Model file for the job. Use its own axes, mm. Face numbers are marked on the shaded views. A direction names the side the tool comes from. Give positions to 0.01 mm unless a question says otherwise; leave off trailing zeros. Write each loop counter-clockwise with the first axis right and the second up, starting at its lowest first coordinate (ties: lowest second). Pieces come first, ordered by that corner, then holes. Notation, with made-up numbers: (38.5, -28.75) - (60.5, -28.75) arc R22 cw to (60.5, -2.75) - close; hole circle Ø5 at (-20.5, 89). An arc over 180 degrees is marked (long way). One line per item, written item: value. Start each with the question number.
(1) Cut at B-B, the plane z = -51. List the corners of the cut face in (x, y).
(2) Probe L1, parallel to Z at x = 23, y = -18; L2, parallel to Z at x = 6.5, y = 14.5; L3, parallel to X at y = -21, z = -52. List the from-to ranges inside material, lowest first.
(3) Cut at A-A, the plane x = 33.25. List the corners of the cut face in (y, z), and give its area (3 significant figures).
(4) Mould opens along Z. For the marked faces 4, 5 and 6 say: pulls with the +Z half, pulls with the -Z half, needs draft (parallel to the pull), parting line crosses it, or undercut.
(5) Cut at C-C, the plane y = 23. List the corners of the cut face in (x, z).
(6) Drop flat-ended pins along their axis: P1, Ø3, axis at x = 5.5, y = 19.5, coming from the +Z side; P2, Ø12, axis at y = -13.5, z = 2.5, coming from the -X side; P3, Ø4, axis at x = 30, y = -21, coming from the -Z side; P4, Ø13, axis at x = 10.5, y = -6.5, coming from the +Z side. Give the stop position or say it passes through.
(7) 3-axis set-ups, long thin cutter, end or side, ignore diameter. For the marked faces 1, 2 and 3: which of +Z, -Z, +X, -X, +Y, -Y reach the whole face in a straight line?
from build123d import *

# Parameters (mm, degrees)
SALIENTE_EXTRUIR1_DEPTH = 42
CROQUIS2_W              = 11
CROQUIS2_H              = 10
SALIENTE_EXTRUIR2_DEPTH = 6
CROQUIS3_R              = 3.25
SALIENTE_EXTRUIR3_DEPTH = 10
CROQUIS4_R              = 9
SALIENTE_EXTRUIR4_DEPTH = 16.5
CROQUIS5_W              = 20
CROQUIS5_H              = 25
SALIENTE_EXTRUIR5_DEPTH = 16
CROQUIS6_R              = 3.5
SALIENTE_EXTRUIR6_DEPTH = 1
REDONDEO2_R             = 4


with BuildPart() as part:
    # Croquis1 → Saliente-Extruir1 (new body)
    with BuildSketch(Plane(origin=(0, 0, 0), x_dir=(0, 0, -1), z_dir=(1, 0, 0))):
        Polygon((21.5, 2.5), (25.5, 2.5), (25.5, -13.5), (21.5, -13.5), (21.5, -41.5), (-21.5, -41.5), (-21.5, -13.5), (-22.5, -13.5), (-22.5, 2.5), (-21.5, 2.5), (-21.5, 41.5), (21.5, 41.5), align=None)
    extrude(amount=SALIENTE_EXTRUIR1_DEPTH)

    # Croquis2 → Saliente-Extruir2 (add)
    with BuildSketch(Plane.XY.offset(21.5)):
        with Locations((21, 36.5)):
            Rectangle(CROQUIS2_W, CROQUIS2_H)
    extrude(amount=SALIENTE_EXTRUIR2_DEPTH)

    # Croquis3 → Saliente-Extruir3 (add)
    with BuildSketch(Plane.XY.offset(22.5)):
        with Locations(Location((33.25, -7.5, 0), (0, 0, 180))):
            Circle(CROQUIS3_R)
    extrude(amount=SALIENTE_EXTRUIR3_DEPTH)

    # Croquis4 → Saliente-Extruir4 (add)
    with BuildSketch(Plane(origin=(0, 0, -25.5), x_dir=(-1, 0, 0), z_dir=(0, 0, -1))):
        with Locations(Location((-16, -8.5, 0), (0, 0, 213.748988596))):
            Circle(CROQUIS4_R)
    extrude(amount=SALIENTE_EXTRUIR4_DEPTH)

    # Croquis5 → Saliente-Extruir5 (add)
    with BuildSketch(Plane(origin=(0, 0, -42), x_dir=(-1, 0, 0), z_dir=(0, 0, -1))):
        with Locations((-16, -12)):
            Rectangle(CROQUIS5_W, CROQUIS5_H)
    extrude(amount=SALIENTE_EXTRUIR5_DEPTH)

    # Croquis6 → Saliente-Extruir6 (add)
    with BuildSketch(Plane(origin=(0, 0, -58), x_dir=(-1, 0, 0), z_dir=(0, 0, -1))):
        with Locations((-16, -8.5)):
            Circle(CROQUIS6_R)
    extrude(amount=SALIENTE_EXTRUIR6_DEPTH)

    # Redondeo2
    # the kernel refuses this fillet: 4 mm, written as the material it takes off along each edge
    with BuildSketch(Plane(origin=(16, -8.5, -59), x_dir=(-1, 0, 0), z_dir=(0, -1, 0))) as redondeo2_piece_1:
        with BuildLine():
            CenterArc((0.854248689, -4), REDONDEO2_R, 48.590377891, 41.409622109)
            Line((0.854248689, 0), (0.854248689, 0.08))
            Line((0.854248689, 0.08), (3.5, 0.08))
            Line((3.5, 0.08), (3.58, 0))
            ThreePointArc((3.58, 0), (3.58, -0.5), (3.552915026, -0.94))
            Line((3.552915026, -0.94), (3.5, -1))
        make_face()
    revolve(axis=Axis((16, -8.5, -59), (0, 0, -1)), mode=Mode.SUBTRACT)


solid = part.part
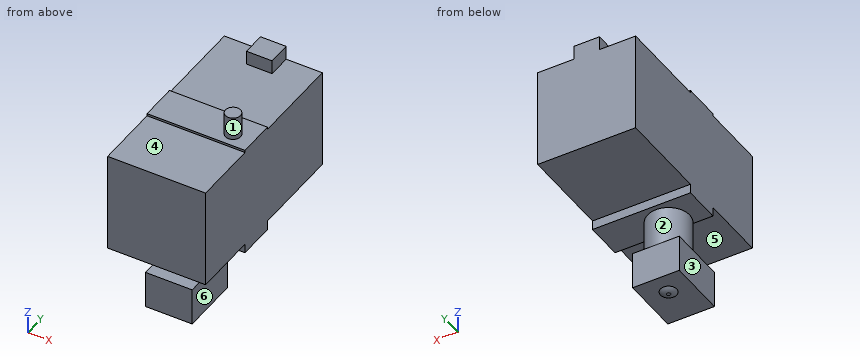
Answers follow:
1. outline: (6, -24.5) - (26, -24.5) - (26, 0.5) - (6, 0.5) - close
2. L1: z = -58 to -42, -21.5 to 21.5
2. L2: z = -21.5 to 21.5
2. L3: x = 6 to 26
3. outline: (-41.5, -21.5) - (-13.5, -21.5) - (-13.5, -25.5) - (2.5, -25.5) - (2.5, -21.5) - (41.5, -21.5) - (41.5, 21.5) - (2.5, 21.5) - (2.5, 22.5) - (-4.25, 22.5) - (-4.25, 32.5) - (-10.75, 32.5) - (-10.75, 22.5) - (-13.5, 22.5) - (-13.5, 21.5) - (-41.5, 21.5) - close
3. area: 3,710 mm²
4. face 4: pulls with the +Z half
4. face 5: undercut
4. face 6: needs draft
5. outline: (0, -21.5) - (42, -21.5) - (42, 21.5) - (0, 21.5) - close
6. P1: stops at z = 21.5
6. P2: stops at x = 0
6. P3: stops at z = -21.5
6. P4: stops at z = 22.5
7. face 1: +Z
7. face 2: none
7. face 3: -Z, -X, +Y, -Y
